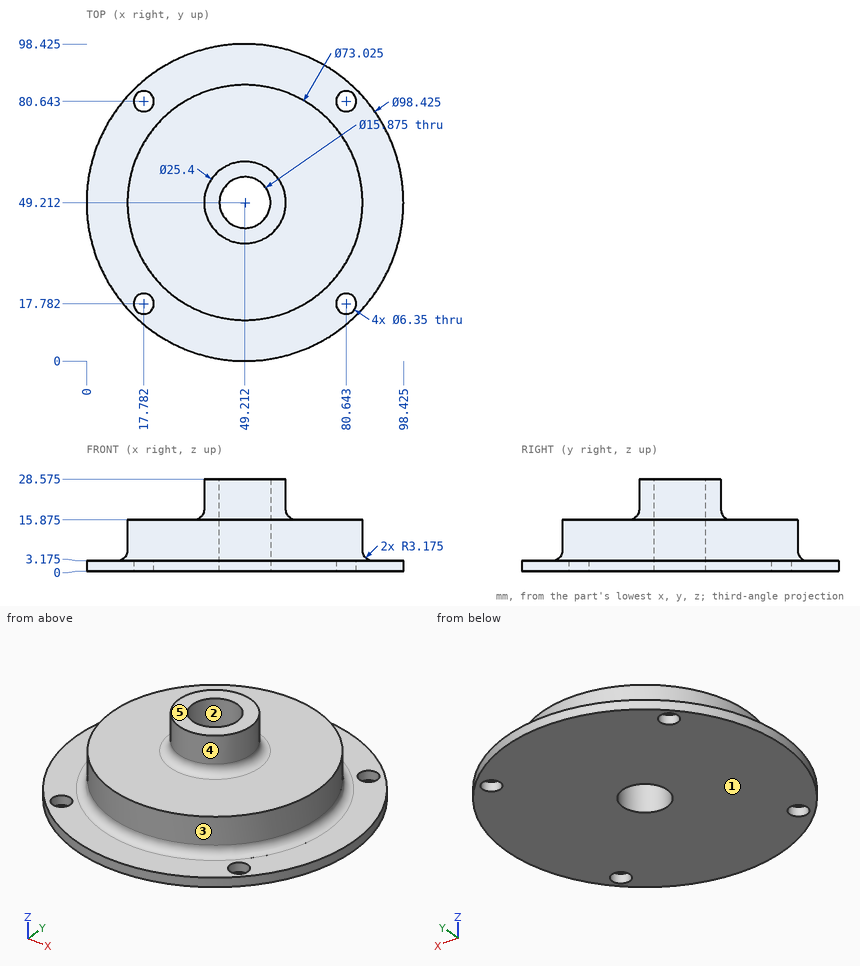
The figure shows three views and two pictorial views of one solid part (mm, origin at its lowest corner). Answer the questions. A direction names the side the tool comes from. Round coordinates to 2 decimals unless told otherwise and drop trailing zeros. One line per item, written item: value.
Item 1: For the marked faces 4 and 5, determine the directions among +Z, -Z, +X, -X, +Y, -Y from which every point of the face is accessible in a straight line to the end or side of a thin tool.
Taken from the geometry:
face 4: +Z
face 5: +Z, +X, -X, +Y, -Y
Item 2: For a pull along X with two mould halves and no side action, classify the marked faces 1, 2 and 3 as released by +X, released by -X, zero draft, split by the parting line, or undercut.
Taken from the geometry:
face 1: zero draft
face 2: undercut
face 3: split by the parting line
Item 3: Given P1, Ø8, axis at x = 63.5, z = 24.5, coming from the +Y side; P2, Ø2, axis at y = 87.5, z = 4, coming from the -X side (1 decimal); P3, Ø1.5, axis at x = 37.5, y = 42, coming from the +Z side (1 decimal), each flat-ended and moving along its own axis, determine where each tip first touches the part or whether it passes through.
Taken from the geometry:
P1: stops at y = 56.66
P2: stops at x = 17.6
P3: stops at z = 17.7
Item 4: Straight lines are drawn through the part: L1, parallel to Z at x = 80.5, y = 39 (1 decimal); L2, parallel to Z at x = 14, y = 82 (1 decimal); L3, parallel to Y at x = 50.5, z = 24 (1 decimal). For each, find the intervals that lie inside material, in ascending order.
Taken from the geometry:
L1: z = 0 to 15.9
L2: z = 0 to 3.2
L3: y = 36.6 to 41.4, 57 to 61.8
